Source: three-view drawing plus pictorial views. Frame: mm from the lowest corner of the part. Give positions to 0.01 mm unless a question says otherwise; leave off trailing zeros. Loops run counter-clockwise (first coordinate to the right, second up) from the corner with the lowest first, then second, coordinate; pieces in that order, holes last.
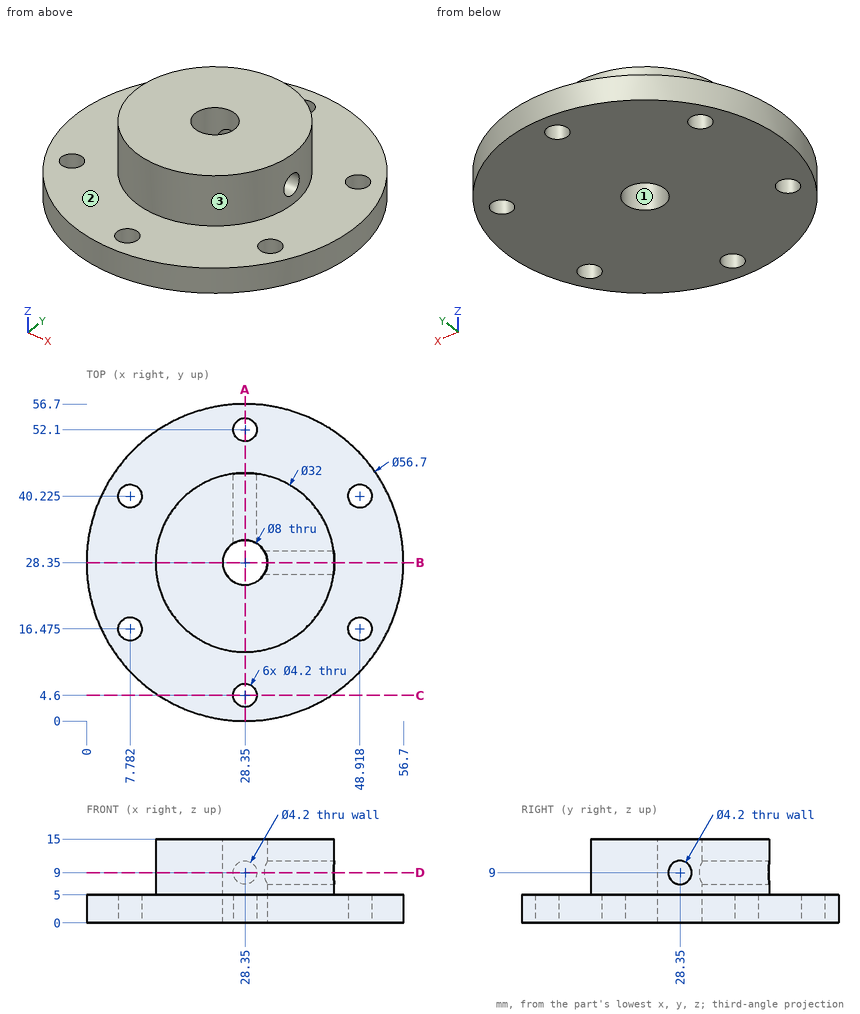
(1) Pin query (flat end, axial travel): pin 1 Ø6.5 at (y, z) = (28.35, 9) entering from +X; pin 2 Ø5.5 at (x, y) = (7.78, 40.23) entering from +Z; pin 3 Ø1.5 at (x, z) = (17, 12.5) entering from +Y (3 decimals). Return the tip coordinate at first contact, or that it passes through.
Values follow:
pin 1: stops at x = 44.35
pin 2: stops at z = 5
pin 3: stops at y = 40.335
(2) Cut plane C-C (y = 4.6). Return the cut outline in (x, z), and give its area (3 significant figures).
Values follow:
outline: (12.87, 0) - (26.25, 0) - (26.25, 5) - (12.87, 5) - close; (30.45, 0) - (43.83, 0) - (43.83, 5) - (30.45, 5) - close
area: 134 mm2
(3) Mould query, pull axis Y, two halves, no side actions, for the marked faces 1, 2 and 3. Classes: +Y half, -Y half, draft (parallel to the pull), parting line (faces both ways), or undercut.
Values follow:
face 1: undercut
face 2: draft
face 3: parting line
(4) Cut plane A-A (x = 28.35). Return the cut outline in (y, z), and give its area (3 significant figures).
Values follow:
outline: (0, 0) - (2.5, 0) - (2.5, 5) - (0, 5) - close; (6.7, 0) - (24.35, 0) - (24.35, 15) - (12.35, 15) - (12.35, 5) - (6.7, 5) - close; (32.35, 0) - (50, 0) - (50, 5) - (44.35, 5) - (44.35, 6.9) - (32.35, 6.9) - close; (32.35, 11.1) - (44.35, 11.1) - (44.35, 15) - (32.35, 15) - close; (54.2, 0) - (56.7, 0) - (56.7, 5) - (54.2, 5) - close
area: 391 mm2
(5) Cut plane B-B (y = 28.35). Return the cut outline in (x, z), and give its area (3 significant figures).
Values follow:
outline: (0, 0) - (24.35, 0) - (24.35, 15) - (12.35, 15) - (12.35, 5) - (0, 5) - close; (32.35, 0) - (56.7, 0) - (56.7, 5) - (44.35, 5) - (44.35, 6.9) - (32.35, 6.9) - close; (32.35, 11.1) - (44.35, 11.1) - (44.35, 15) - (32.35, 15) - close
area: 433 mm2
(6) Cut plane D-D (z = 9). Return the cut outline in (x, y), and give its area (3 significant figures).
Values follow:
outline: (26.25, 31.75) - (26.25, 44.21) arc R16 ccw (long way) to (44.21, 26.25) - (31.75, 26.25) arc R4 cw (long way) to start; (30.45, 31.75) arc R4 cw to (31.75, 30.45) - (44.21, 30.45) arc R16 ccw to (30.45, 44.21) - close
area: 652 mm2
(7) Ray query, probe 1 along Y at (x, z) = (28.35, 2.2); probe 2 along Z at (x, y) = (42, 48); probe 3 along X at (y, z) = (27, 1) (1 decimal). Return the intervals inside material, ascending.
Values follow:
probe 1: y = 0 to 2.5, 6.7 to 24.35, 32.35 to 50, 54.2 to 56.7
probe 2: z = 0 to 5
probe 3: x = 0 to 24.6, 32.1 to 56.7
